The model under review builds one solid part; all positions refer to its coordinate system, in mm. A direction names the side the tool comes from. Give positions to 0.01 mm unless a question says otherwise; leave off trailing zeros. Order: outer loops, then holes, each group sorted by start corner. A loop starts at its lowest first (then second) coordinate and runs counter-clockwise, first axis right, second up. Notation, with made-up numbers: (13, -24) - (65, -24) arc R23 ccw to (65, -6) - close; hole circle Ø8 at (63, -15). An arc over 180 degrees is marked (long way). Put each result on its own line as item: value.
```python
from build123d import *

# Parameters (mm, degrees)
SKETCH1_R           = 13.8
BOSS_EXTRUDE1_DEPTH = 38
BOSS_EXTRUDE2_START = -34.5
BOSS_EXTRUDE2_DEPTH = 21
SKETCH3_R           = 5
BOSS_EXTRUDE3_DEPTH = 2.8
SKETCH4_R           = 13.5
CUT_EXTRUDE1_DEPTH  = 1.2
SKETCH5_R           = 5
BOSS_EXTRUDE4_DEPTH = 3.5
SKETCH6_R           = 1.15
BOSS_EXTRUDE5_DEPTH = 5.8
SKETCH7_R           = 1.15
BOSS_EXTRUDE6_DEPTH = 8
SKETCH8_R           = 1.25
CUT_EXTRUDE2_DEPTH  = 8


with BuildPart() as part:
    # Sketch1 → Boss-Extrude1 (new body)
    with BuildSketch(Plane.XY):
        Circle(SKETCH1_R)
    extrude(amount=BOSS_EXTRUDE1_DEPTH)

    # Sketch2 → Boss-Extrude2 (add)
    with BuildSketch(Plane.XY.offset(38).offset(BOSS_EXTRUDE2_START)):
        with BuildLine():
            Line((-1.458768031, 14.677687006), (-1.36481348, 13.732344453))
            ThreePointArc((-1.36481348, 13.732344453), (3.145567943, -13.436718436), (-4.872500867, 12.911186441))
            Line((-4.872500867, 12.911186441), (-5.207926651, 13.8))
            ThreePointArc((-5.207926651, 13.8), (3.362110664, -14.361709922), (-1.458768031, 14.677687006))
        make_face()
    extrude(amount=BOSS_EXTRUDE2_DEPTH)

    # Sketch3 → Boss-Extrude3 (add)
    with BuildSketch(Plane(origin=(0, 0, 0), x_dir=(-1, 0, 0), z_dir=(0, 0, -1))):
        Circle(SKETCH3_R)
    extrude(amount=BOSS_EXTRUDE3_DEPTH)

    # Sketch4 → Cut-Extrude1 (cut)
    with BuildSketch(Plane.XY.offset(38)):
        Circle(SKETCH4_R)
    extrude(amount=-CUT_EXTRUDE1_DEPTH, mode=Mode.SUBTRACT)

    # Sketch5 → Boss-Extrude4 (add)
    with BuildSketch(Plane.XY.offset(36.8)):
        Circle(SKETCH5_R)
    extrude(amount=BOSS_EXTRUDE4_DEPTH)

    # Sketch6 → Boss-Extrude5 (add)
    with BuildSketch(Plane.XY.offset(40.3)):
        Circle(SKETCH6_R)
    extrude(amount=BOSS_EXTRUDE5_DEPTH)

    # Sketch7 → Boss-Extrude6 (add)
    with BuildSketch(Plane(origin=(0, 0, -2.8), x_dir=(-1, 0, 0), z_dir=(0, 0, -1))):
        Circle(SKETCH7_R)
    extrude(amount=BOSS_EXTRUDE6_DEPTH)

    # Sketch8 → Cut-Extrude2 (cut)
    with BuildSketch(Plane(origin=(0, 0, 0), x_dir=(-1, 0, 0), z_dir=(0, 0, -1))):
        with Locations((-7.789401992, 1.823517648)):
            Circle(SKETCH8_R)
        with Locations((7.789401992, -1.823517648)):
            Circle(SKETCH8_R)
    extrude(amount=-CUT_EXTRUDE2_DEPTH, mode=Mode.SUBTRACT)


solid = part.part
```
(1) Wall thickness on L1, parallel to Y at x = 0, z = 37.25; L2, parallel to Z at x = -6.25, y = 11; L3, parallel to Z at x = -13.5, y = -2: over which ranges is each line inside the solid? List them lowest first.
The answers:
L1: -13.8 to -13.5, -5 to 5, 13.5 to 13.8
L2: 0 to 36.8
L3: 0 to 38
(2) Take a section at C-C, the plane y = 10. Write out the cut boundary in (x, z), then the cut area to 3 significant figures.
The answers:
outline: (-10.84, 3.5) - (-9.51, 3.5) - (-9.51, 0) - (9.51, 0) - (9.51, 3.5) - (10.84, 3.5) - (10.84, 24.5) - (9.51, 24.5) - (9.51, 38) - (9.07, 38) - (9.07, 36.8) - (-9.07, 36.8) - (-9.07, 38) - (-9.51, 38) - (-9.51, 24.5) - (-10.84, 24.5) - close
area: 757 mm^2
(3) For faces 4 (the flat face through (8, 2, 8)), 5 (the cylindrical face through (-0.91, -0.7, 43.16)), 6 (the cylindrical face through (-1.796, 13.683, 22.956)), list the 3-axis set-ups (+Z, -Z, +X, -X, +Y, -Y) from which the entire face can be reached by the end or side of a thin tool; tool diameter is ignored.
The answers:
face 4: -Z
face 5: +Z
face 6: none
(4) Clearance check with flat-ended pins moving along their axes: pin 1 Ø12 at (x, y) = (8, -11) entering from +Z; pin 2 Ø12 at (x, z) = (0.5, 31.5) entering from -Y; pin 3 Ø3 at (x, y) = (-7.79, -1.82) entering from -Z. State where each tip first meets the part, or that it passes through.
The answers:
pin 1: z = 38
pin 2: y = -13.8
pin 3: z = 0
(5) The part is to be moulded in two halves that separate along X. For faces 1 (the cylindrical face through (-2.93, -13.18, 37.41)), 2 (the flat face through (6, 0, 0)), 3 (the cylindrical face through (2.75, -14.49, 13.85)), say which applies: pulls with the +X half, pulls with the -X half, needs draft (parallel to the pull), parting line crosses it, or undercut.
The answers:
face 1: undercut
face 2: needs draft
face 3: parting line crosses it
(6) Take a section at D-D, the plane x = 3. Write out the cut boundary in (y, z).
The answers:
outline: (-14.44, 3.5) - (-13.47, 3.5) - (-13.47, 0) - (-4, 0) - (-4, -2.8) - (4, -2.8) - (4, 0) - (13.47, 0) - (13.47, 3.5) - (14.44, 3.5) - (14.44, 24.5) - (13.47, 24.5) - (13.47, 38) - (13.16, 38) - (13.16, 36.8) - (4, 36.8) - (4, 40.3) - (-4, 40.3) - (-4, 36.8) - (-13.16, 36.8) - (-13.16, 38) - (-13.47, 38) - (-13.47, 24.5) - (-14.44, 24.5) - close
